CAD build for the part. Positions are in the model's coordinates, mm. Round coordinates to 2 decimals unless told otherwise and drop trailing zeros. Order: outer loops, then holes, each group sorted by start corner. A loop starts at its lowest first (then second) coordinate and runs counter-clockwise, first axis right, second up. Notation, with made-up numbers: (9.5, 58) -> (34.5, 58) arc R34 ccw to (34.5, 89) -> close; hole circle Ø1 at (-16.5, 3). An arc over 180 degrees is marked (long way). Return JSON: item names as keys, results as strings. Group by question number.
Q1. Cut at C-C (y = 88.9). Write the cut outline in (x, z) (3 decimals), then the cut area to 3 significant figures.
Q2. Cut at B-B (z = 9.25). Count the separate pieces of the cut face and the enclosed holes in it, then the cut area to 3 significant figures.
Q3. Flat gauge pins, fed straight in: pin 1 (5.5 mm diameter, centred on x = 0, y = -88.9, fed in from -Z); pin 2 (1 mm diameter, centred on y = -77, z = 7.5, fed in from -X). Where does each tip first touch, or does it go through?
Q4. Probe line 1 along X through (y, z) = (-139.7, 3.5); line 2 along Y through (x, z) = (50.8, 4); line 3 along Y through (x, z) = (0, 10.25) (3 decimals). List the from-to ranges inside material, lowest first.
Q5. Cut at A-A (y = -88.9). Write the cut outline in (x, z) (3 decimals), then the cut area to 3 significant figures.
Q6. Cut at D-D (x = -63.5). Write the cut outline in (y, z) (3 decimals), then the cut area to 3 significant figures.
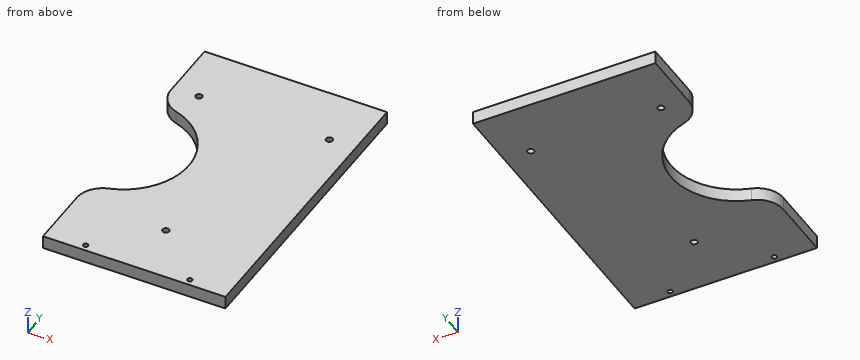
from build123d import *

# Parameters (mm, degrees)
F0_R     = 3.175
F1_DEPTH = 12.7
F2_R     = 25.4
F3_R     = 2.38125
F4_DEPTH = 12.701


with BuildPart() as f1:
    # F0 (on Top) → F1 (new body)
    with BuildSketch(Plane.XY):
        with BuildLine():
            Line((88.9, -146.05), (88.9, 146.05))
            Line((88.9, 146.05), (-88.9, 146.05))
            Line((-88.9, 146.05), (-88.9, 63.5))
            ThreePointArc((-88.9, 63.5), (-25.4, 0), (-88.9, -63.5))
            Line((-88.9, -63.5), (-88.9, -146.05))
            Line((-88.9, -146.05), (88.9, -146.05))
        make_face()
        with Locations((0, -88.9)):
            Circle(F0_R, mode=Mode.SUBTRACT)
        with Locations((-63.5, 88.9)):
            Circle(F0_R, mode=Mode.SUBTRACT)
        with Locations((63.5, 88.9)):
            Circle(F0_R, mode=Mode.SUBTRACT)
    extrude(amount=F1_DEPTH)

    # F2
    f2_edges = [f1.edges().sort_by_distance(p)[0] for p in [
        (-88.9, -63.5, 6.35),
        (-88.9, 63.5, 6.35),
    ]]
    fillet(f2_edges, radius=F2_R)

    # F3 (on face) → F4 (cut, through all)
    with BuildSketch(Plane.XY.offset(12.7)):
        with Locations((-50.8, -139.7)):
            Circle(F3_R)
        with Locations((50.8, -139.7)):
            Circle(F3_R)
    extrude(amount=-F4_DEPTH, mode=Mode.SUBTRACT)


solid = f1.part
Solution:
{
 "1": {"outline": "(-88.9, 0) -> (-66.675, 0) -> (-66.675, 12.7) -> (-88.9, 12.7) -> close; (-60.325, 0) -> (60.325, 0) -> (60.325, 12.7) -> (-60.325, 12.7) -> close; (66.675, 0) -> (88.9, 0) -> (88.9, 12.7) -> (66.675, 12.7) -> close", "area": "2,100 mm²"},
 "2": {"separate pieces": "1", "enclosed holes": "5", "area": "45,300 mm²"},
 "3": {"pin 1": "passes through", "pin 2": "stops at x = -87.71"},
 "4": {"line 1": "x = -88.9 to -53.18, -48.42 to 48.42, 53.18 to 88.9", "line 2": "y = -146.05 to -142.08, -137.32 to 146.05", "line 3": "y = -146.05 to -92.075, -85.725 to 146.05"},
 "5": {"outline": "(-88.9, 0) -> (-3.175, 0) -> (-3.175, 12.7) -> (-88.9, 12.7) -> close; (3.175, 0) -> (88.9, 0) -> (88.9, 12.7) -> (3.175, 12.7) -> close", "area": "2,180 mm²"},
 "6": {"outline": "(-146.05, 0) -> (-58.199, 0) -> (-58.199, 12.7) -> (-146.05, 12.7) -> close; (58.199, 0) -> (85.725, 0) -> (85.725, 12.7) -> (58.199, 12.7) -> close; (92.075, 0) -> (146.05, 0) -> (146.05, 12.7) -> (92.075, 12.7) -> close", "area": "2,150 mm²"}
}
